from build123d import *

# Parameters (mm, degrees)
SKETCH_1_W      = 100
SKETCH_1_H      = 100
SKETCH_1_R      = 1.5
EXTRUDE_1_DEPTH = 5
FILLET_1_R      = 20


with BuildPart() as part:
    # 草图1 → 凸台-拉伸1 (new body)
    with BuildSketch(Plane(origin=(0, 0, 0), x_dir=(1, 0, 0), z_dir=(0, 1, 0))):
        Rectangle(SKETCH_1_W, SKETCH_1_H)
        with Locations((-35, 35)):
            Circle(SKETCH_1_R, mode=Mode.SUBTRACT)
        with Locations((35, 35)):
            Circle(SKETCH_1_R, mode=Mode.SUBTRACT)
        with Locations((35, -35)):
            Circle(SKETCH_1_R, mode=Mode.SUBTRACT)
        with Locations((-35, -35)):
            Circle(SKETCH_1_R, mode=Mode.SUBTRACT)
        with Locations((-10, 10)):
            Circle(SKETCH_1_R, mode=Mode.SUBTRACT)
        with Locations((10, 10)):
            Circle(SKETCH_1_R, mode=Mode.SUBTRACT)
        with Locations((10, -10)):
            Circle(SKETCH_1_R, mode=Mode.SUBTRACT)
        with Locations((-10, -10)):
            Circle(SKETCH_1_R, mode=Mode.SUBTRACT)
    extrude(amount=EXTRUDE_1_DEPTH)

    # 圆角1
    fillet_1_edges = [part.edges().sort_by_distance(p)[0] for p in [
        (-50, 2.5, -50),
        (50, 2.5, -50),
        (50, 2.5, 50),
        (-50, 2.5, 50),
    ]]
    fillet(fillet_1_edges, radius=FILLET_1_R)


solid = part.part
Geometry check sheet. Reference: the model listing, model coordinates, mm. Round coordinates to 2 decimals unless told otherwise and drop trailing zeros. Order: outer loops, then holes, each group sorted by start corner. A loop starts at its lowest first (then second) coordinate and runs counter-clockwise, first axis right, second up. Notation, with made-up numbers: M 72,-21.75 L 106,-21.75 A11 ccw 106,-10.75 Z; hole C 30.25,61 d2. An arc over 180 degrees is marked long. Answer in a Markdown table with one row per item. Add a question column.
Item 1: Sectioned sample at C-C, the plane z = -10. Enter the section's corners in (x, y), plus the area to 3 significant figures.
Item 2: Material ranges on L1, parallel to X at y = 3.65, z = -10; L2, parallel to Z at x = -9, y = 0.7, recorded low to high. Write a range as [from, to].
Item 3: Sectioned sample at D-D, the plane z = 42.5. Enter the section's corners in (x, y).
Item 4: Sectioned sample at B-B, the plane y = 2.75. State how many separate pieces and enclosed holes the cut face has, plus the area to 3 significant figures.
Item 5: Sectioned sample at A-A, the plane x = -10. Enter the section's corners in (y, z).
Item 6: Draft check along X on faces 1 (the face through (-1, 5, -1)), 2 (the face through (-11.2, 2.5, 10.9)), 3 (the face through (-44.297, 2.535, -43.986)). Enter one of: released by +X, released by -X, zero draft, split by the parting line, or undercut.
Filled in:
| question | item | result |
|---|---|---|
| 1 | outline | M -50,0 L -11.5,0 L -11.5,5 L -50,5 Z; M -8.5,0 L 8.5,0 L 8.5,5 L -8.5,5 Z; M 11.5,0 L 50,0 L 50,5 L 11.5,5 Z |
| 1 | area | 470 mm² |
| 2 | L1 | x = [-50, -11.5], [-8.5, 8.5], [11.5, 50] |
| 2 | L2 | z = [-50, -11.12], [-8.88, 8.88], [11.12, 50] |
| 3 | outline | M -45.61,0 L 45.61,0 L 45.61,5 L -45.61,5 Z |
| 4 | separate pieces | 1 |
| 4 | enclosed holes | 8 |
| 4 | area | 9,600 mm² |
| 5 | outline | M 0,-50 L 5,-50 L 5,-11.5 L 0,-11.5 Z; M 0,-8.5 L 5,-8.5 L 5,8.5 L 0,8.5 Z; M 0,11.5 L 5,11.5 L 5,50 L 0,50 Z |
| 6 | face 1 | zero draft |
| 6 | face 2 | undercut |
| 6 | face 3 | released by -X |
